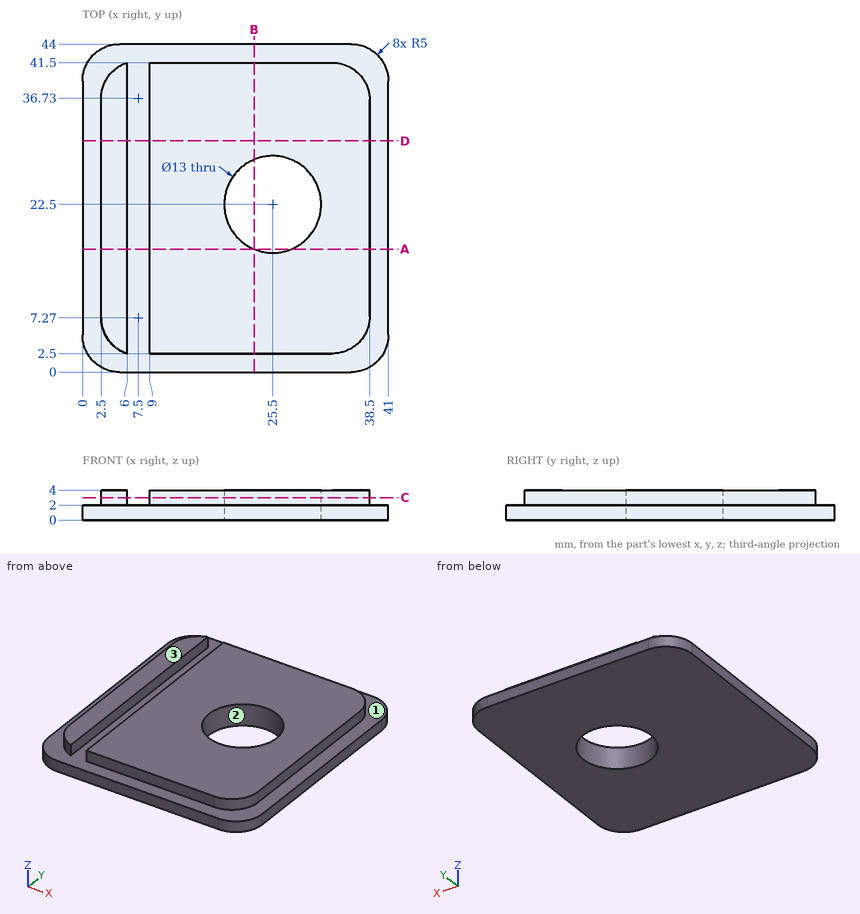
Answer from the drawing. Dimensions are ordinates in mm from the lowest x, y and z of the part. Coordinates: 2 decimals unless noted, no trailing zeros. Write each loop counter-clockwise with the first axis right and the second up, starting at its lowest first coordinate (ties: lowest second). Pieces come first, ordered by that corner, then holes. Notation, with made-up numbers: M 78.5,28.25 L 89.5,28.25 A9 cw 89.5,37.25 Z; hole C -7.75,-5.75 d4. An arc over 180 degrees is marked long. Write item = value, one per line.
1. Determine the mould class of the marked faces 1, 2 and 3 for opening direction X: released by +X, released by -X, zero draft, split by the parting line, or undercut.
Solution:
face_1 = undercut
face_2 = undercut
face_3 = zero draft
2. Straight lines are drawn through the part: line 1 (X direction, y = 34.5, z = 2.3); line 2 (Y direction, x = 25.5, z = 2.75); line 3 (Y direction, x = 25.5, z = 1.4). For each, find the intervals that lie inside material, in ascending order. Write a range as from..to.
Solution:
line_1 = 2.5..6, 9..38.5
line_2 = 2.5..16, 29..41.5
line_3 = 0..16, 29..44
3. Flat-ended cylindrical pins translate along their axes: pin 1 (1 mm diameter, centred on x = 16, z = 3, fed in from -Y); pin 2 (3 mm diameter, centred on x = 32.5, y = 22, fed in from -Z); pin 3 (1.6 mm diameter, centred on y = 23, z = 3, fed in from -X); pin 4 (1.6 mm diameter, centred on x = 24.5, z = 3.5, fed in from +Y). Find the tip coordinate at first contact, or state that the pin passes through.
Solution:
pin_1 = 2.5
pin_2 = 0
pin_3 = 2.5
pin_4 = 41.5
4. The part is cut by section C-C (z = 3). Determine the outline of the cut face in (x, y), then the cut area to 3 significant figures.
Solution:
outline = M 2.5,7.27 A5 ccw 6,2.5 L 6,41.5 A5 ccw 2.5,36.73 Z; M 9,2.5 L 33.5,2.5 A5 ccw 38.5,7.5 L 38.5,36.5 A5 ccw 33.5,41.5 L 9,41.5 Z; hole C 25.5,22.5 d13
area = 1,130 mm2
5. The part is cut by section B-B (x = 23). Determine the outline of the cut face in (y, z).
Solution:
outline = M 0,0 L 16.5,0 L 16.5,4 L 2.5,4 L 2.5,2 L 0,2 Z; M 28.5,0 L 44,0 L 44,2 L 41.5,2 L 41.5,4 L 28.5,4 Z
6. The part is cut by section A-A (y = 16.5). Determine the outline of the cut face in (x, z), then the cut area to 3 significant figures.
Solution:
outline = M 0,0 L 23,0 L 23,4 L 9,4 L 9,2 L 6,2 L 6,4 L 2.5,4 L 2.5,2 L 0,2 Z; M 28,0 L 41,0 L 41,2 L 38.5,2 L 38.5,4 L 28,4 Z
area = 128 mm2
7. The part is cut by section D-D (y = 31). Determine the outline of the cut face in (x, z).
Solution:
outline = M 0,0 L 41,0 L 41,2 L 38.5,2 L 38.5,4 L 9,4 L 9,2 L 6,2 L 6,4 L 2.5,4 L 2.5,2 L 0,2 Z
